Source: CAD feature listing. Evaluate the final solid. Frame: model axes, mm. A direction names the side the tool comes from. Round coordinates to 2 decimals unless told otherwise and drop trailing zeros. Order: outer loops, then holes, each group sorted by start corner. A loop starts at its lowest first (then second) coordinate and runs counter-clockwise, first axis right, second up. Notation, with made-up numbers: (-11.5, -31.75) -> (5.5, -31.75) arc R37 cw to (5.5, 7.25) -> close; hole circle Ø7 at (-33, -19). An arc over 180 degrees is marked (long way). Use a Markdown table: item, result. Add a question column.
```python
from build123d import *

# Parameters (mm, degrees)
SKETCH1_W           = 140
SKETCH1_H           = 60
BOSS_EXTRUDE1_DEPTH = 160
SHELL1_T            = -5
SKETCH2_R           = 2.6
SKETCH2_R_2         = 2.1
SKETCH2_W           = 42
SKETCH2_H           = 25
CUT_EXTRUDE1_DEPTH  = 161
FILLET1_R           = 10


with BuildPart() as part:
    # Sketch1 → Boss-Extrude1 (new body)
    with BuildSketch(Plane.XY):
        with Locations((-70, 30)):
            Rectangle(SKETCH1_W, SKETCH1_H)
    extrude(amount=BOSS_EXTRUDE1_DEPTH)

    # Shell1
    shell1_openings = [part.faces().sort_by_distance(p)[0] for p in [
        (-70, 60, 80),
    ]]
    offset(amount=SHELL1_T, openings=shell1_openings, kind=Kind.INTERSECTION)

    # Sketch2 → Cut-Extrude1 (cut, through all)
    with BuildSketch(Plane.XY.offset(160)):
        with Locations((-127.5, 50)):
            Circle(SKETCH2_R)
        with Locations((-127.5, 10)):
            Circle(SKETCH2_R)
        with Locations((-12.5, 10)):
            Circle(SKETCH2_R)
        with Locations((-12.5, 50)):
            Circle(SKETCH2_R)
        with Locations((-130, 35)):
            Circle(SKETCH2_R_2)
        with Locations((-130, 25)):
            Circle(SKETCH2_R_2)
        with Locations((-82, 25)):
            Circle(SKETCH2_R_2)
        with Locations((-82, 35)):
            Circle(SKETCH2_R_2)
        with Locations((-58, 25)):
            Circle(SKETCH2_R_2)
        with Locations((-58, 35)):
            Circle(SKETCH2_R_2)
        with Locations((-10, 25)):
            Circle(SKETCH2_R_2)
        with Locations((-10, 35)):
            Circle(SKETCH2_R_2)
        with Locations((-106, 30)):
            Rectangle(SKETCH2_W, SKETCH2_H)
        with Locations((-34, 30)):
            Rectangle(SKETCH2_W, SKETCH2_H)
    extrude(amount=-CUT_EXTRUDE1_DEPTH, mode=Mode.SUBTRACT)

    # Fillet1
    fillet1_edges = [part.edges().sort_by_distance(p)[0] for p in [
        (0, 0, 80),
        (-140, 0, 80),
    ]]
    fillet(fillet1_edges, radius=FILLET1_R)


solid = part.part
```
1) Draft query along X for faces 4 (the flat face through (-138, 60, 80)), 5 (the flat face through (-34, 17.5, 158)), 6 (the cylindrical face through (-137.15, 3.01, 81.12)), 7 (the flat face through (0, 35, 79)). Return one class per face: pulls with the +X half, pulls with the -X half, needs draft (parallel to the pull), parting line crosses it, or undercut.
2) Section B-B on y = 55.5. Output: boundary loops of the cut face in (x, z), then the cut area to 3 significant figures.
3) Section D-D on z = 57. Output: boundary loops of the cut face in (x, y).
4) Reachability of faces 1 (the flat face through (-85, 30, 158)), 2 (the flat face through (-135, 32, 79)), 3 (the flat face through (-71, 30, 160)) from +Z, -Z, +X, -X, +Y, -Y: full face, straight path, thin tool, end or side. Return the list, or none.
5) Section C-C on y = 21. Output: boundary loops of the cut face in (x, z), then the cut area to 3 significant figures.
6) Line query: probe 1 along X at (y, z) = (40, 34); probe 2 along Z at (x, y) = (-80, 15); probe 3 along Y at (x, z) = (-82, 158.1). Output: solid intervals per line, ascending. Write a range as from..to.
7) Section A-A on x = -109. Output: boundary loops of the cut face in (y, z).
8) First-contact query: pin 1 Ø4 at (x, y) = (-130, 35) entering from -Z; pin 2 Ø3 at (x, z) = (-84.5, 62) entering from +Y. Flat tips, straight axial feed; report the tip coordinate or a pass-through.
Conclusion:
| question | item | result |
|---|---|---|
| 1 | face 4 | needs draft |
| 1 | face 5 | undercut |
| 1 | face 6 | pulls with the -X half |
| 1 | face 7 | pulls with the +X half |
| 2 | outline | (-140, 0) -> (0, 0) -> (0, 160) -> (-140, 160) -> close; hole (-135, 5) -> (-5, 5) -> (-5, 155) -> (-135, 155) -> close |
| 2 | area | 2,900 mm^2 |
| 3 | outline | (-140, 10) arc R10 ccw to (-130, 0) -> (-10, 0) arc R10 ccw to (0, 10) -> (0, 60) -> (-5, 60) -> (-5, 5) -> (-135, 5) -> (-135, 60) -> (-140, 60) -> close |
| 4 | face 1 | +Z, -Z |
| 4 | face 2 | +Y |
| 4 | face 3 | +Z, +X, -X, +Y, -Y |
| 5 | outline | (-140, 0) -> (-127, 0) -> (-127, 5) -> (-135, 5) -> (-135, 155) -> (-127, 155) -> (-127, 160) -> (-140, 160) -> close; (-85, 0) -> (-55, 0) -> (-55, 5) -> (-85, 5) -> close; (-85, 155) -> (-55, 155) -> (-55, 160) -> (-85, 160) -> close; (-13, 0) -> (0, 0) -> (0, 160) -> (-13, 160) -> (-13, 155) -> (-5, 155) -> (-5, 5) -> (-13, 5) -> close |
| 5 | area | 2,060 mm^2 |
| 6 | probe 1 | x = -140..-135, -5..0 |
| 6 | probe 2 | z = 0..5, 155..160 |
| 6 | probe 3 | y = 0..22.9, 27.1..32.9, 37.1..60 |
| 7 | outline | (0, 0) -> (17.5, 0) -> (17.5, 5) -> (5, 5) -> (5, 155) -> (17.5, 155) -> (17.5, 160) -> (0, 160) -> close; (42.5, 0) -> (60, 0) -> (60, 5) -> (42.5, 5) -> close; (42.5, 155) -> (60, 155) -> (60, 160) -> (42.5, 160) -> close |
| 8 | pin 1 | passes through |
| 8 | pin 2 | stops at y = 5 |
